CAD build for the part. Positions are in the model's coordinates, mm. A direction names the side the tool comes from. Round coordinates to 2 decimals unless told otherwise and drop trailing zeros. Order: outer loops, then holes, each group sorted by start corner. A loop starts at its lowest first (then second) coordinate and runs counter-clockwise, first axis right, second up. Notation, with made-up numbers: M 55.25,50 L 94.25,50 A27 cw 94.25,81 Z; hole C 56.25,23.25 d2. An arc over 180 degrees is marked long. Put each result on its own line as item: value.
```python
from build123d import *

# Parameters (mm, degrees)
PAD002_DEPTH      = 20
CYLINDER017_R     = 1.4
CYLINDER017_DEPTH = 10
ARRAY014_X_COUNT  = 2
ARRAY014_X_PITCH  = 66
BOX031_W          = 70.5
BOX031_H          = 2
BOX031_DEPTH      = 25.4


with BuildPart() as body003:
    # Sketch003 → Pad002 (new body, symmetric)
    with BuildSketch(Plane.YZ):
        with BuildLine():
            Line((78.762321, 19.834602), (78.762321, 11.356619))
            add(Edge.make_bspline(
                [(78.762321, 11.356619), (74.77858, 14.475335), (71.96254, 15.481066), (69.448204, 16.486797), (65.425285, 17.090239), (56.273132, 16.18508), (52.278152, 12.648025)],
                knots=[0, 0, 0, 0, 0.25, 0.5, 0.75, 1, 1, 1, 1], degree=3))
            ThreePointArc((52.278152, 12.648025), (47.975835, 15.871458), (51.608182, 19.834602))
            Line((51.608182, 19.834602), (78.762321, 19.834602))
        make_face()
    extrude(amount=PAD002_DEPTH, both=True)


with BuildPart() as battery_cover_screw_hole_array:
    # Cylinder017 → Cylinder017 (new body)
    with BuildSketch(Plane(origin=(-33, 86, 7), x_dir=(1, 0, 0), z_dir=(0, -1, 0))):
        Circle(CYLINDER017_R)
    extrude(amount=CYLINDER017_DEPTH)

    # Array014 X: battery cover screw hole array ×2


with BuildPart() as battery_cover_screw_hole_array_1:
    add(battery_cover_screw_hole_array.part)
    with Locations(*[(i * ARRAY014_X_PITCH, 0, 0) for i in range(1, ARRAY014_X_COUNT)]):
        add(battery_cover_screw_hole_array.part)


with BuildPart() as battery_cover_plate_fusion:
    # Box031 → Box031 (new body)
    with BuildSketch(Plane(origin=(-35.25, 78, -4.7), x_dir=(1, 0, 0), z_dir=(0, 0, 1))):
        with Locations((35.25, 1)):
            Rectangle(BOX031_W, BOX031_H)
    extrude(amount=BOX031_DEPTH)

    # Cut002003008: cut battery cover screw hole array
    add(battery_cover_screw_hole_array_1.part, mode=Mode.SUBTRACT)

    # Fusion005004008: union Body003
    add(body003.part)


solid = battery_cover_plate_fusion.part
```
Item 1: Probe line 1 along X through (y, z) = (79.1, 7); line 2 along Z through (x, y) = (33, 78.6); line 3 along Y through (x, z) = (12.5, 9.75). List the from-to ranges inside material, lowest first. Write a range as [from, to].
Answers below:
line 1: [-35.25, -34.4], [-31.6, 31.6], [34.4, 35.25]
line 2: [-4.7, 5.6], [8.4, 20.7]
line 3: [78, 80]
Item 2: Tool access for faces 1 (the flat face through (0, 80, 8)), 2 (the flat face through (20, 63, 17)), 3 (the flat face through (0, 65, 19.835)): list every direction of +Z, -Z, +X, -X, +Y, -Y with a clear straight run to the whole face (end or side of a thin tool).
Answers below:
face 1: +Z, -Z, +X, -X, +Y
face 2: +Z, -Z, +X, -Y
face 3: +Z, +X, -X, -Y
Item 3: Band-saw the part on C-C on x = 23. Give the cut face in (y, z), and give its area (3 significant figures).
Answers below:
outline: M 78,-4.7 L 80,-4.7 L 80,20.7 L 78,20.7 Z
area: 50.8 mm²
Item 4: Mould opens along X. For faces 4 (the cylindrical face through (0.28, 47.985, 15.787)), 5 (the cylindrical face through (31.6, 79.01, 7.06)), 6 (the flat face through (-20, 63, 17)) say: pulls with the +X half, pulls with the -X half, needs draft (parallel to the pull), parting line crosses it, or undercut.
Answers below:
face 4: needs draft
face 5: undercut
face 6: pulls with the -X half
Item 5: Band-saw the part on A-A on x = -33. Give the cut face in (y, z).
Answers below:
outline: M 78,-4.7 L 80,-4.7 L 80,5.6 L 78,5.6 Z; M 78,8.4 L 80,8.4 L 80,20.7 L 78,20.7 Z
Item 6: Band-saw the part on B-B on z = 7. Give the cut face in (x, y), and give its area (3 significant figures).
Answers below:
outline: M -35.25,78 L -34.4,78 L -34.4,80 L -35.25,80 Z; M -31.6,78 L 31.6,78 L 31.6,80 L -31.6,80 Z; M 34.4,78 L 35.25,78 L 35.25,80 L 34.4,80 Z
area: 130 mm²
Item 7: Band-saw the part on D-D on z = -0.5. Give the cut face in (x, y), and give its area (3 significant figures).
Answers below:
outline: M -35.25,78 L 35.25,78 L 35.25,80 L -35.25,80 Z
area: 141 mm²
Item 8: Pin check, flat tips, straight feed: P1, Ø1, axis at x = -13, z = 18, coming from the -Y side; P2, Ø12, axis at y = 56.5, z = 15, coming from the +X side; P3, Ø1.5, axis at x = 11.5, y = 68, coming from the +Z side. Stop position of each tip, or through.
Answers below:
P1: y = 48.2
P2: x = 20
P3: z = 19.83
